```python
from build123d import *

# Parameters (mm, degrees)
CUT_EXTRUDE1_DEPTH      = 164.536310953
CUT_EXTRUDE1_DEPTH_BACK = 164.536310953
SKETCH2_R               = 6.05
SCALE1_SCALE            = 0.25


with BuildPart() as part:
    # Sketch1 → Revolve1 (revolve)
    with BuildSketch(Plane(origin=(0, 0, 0), x_dir=(0, 0, -1), z_dir=(1, 0, 0))):
        Polygon((-60, -15.260894059), (-60, -94.260894059), (-101.25, -94.260894059), (-101.25, -107.260894059), (-101.25, -115.260894059), (-54, -115.260894059), (-54, -94.260894059), (-34.1, -94.260894059), (-30, -94.160894059), (-30, -36.260894059), (-54, -36.260894059), (-54, -15.260894059), align=None)
    revolve(axis=Axis((0, 150, 0), (0, -1, 0)))

    # Sketch2 → Cut-Extrude1 (cut, two sides: drawn at the far end of the back side and taken through both)
    with BuildSketch(Plane(origin=(0, -94.260894059, 0), x_dir=(1, 0, 0), z_dir=(0, 1, 0)).offset(-CUT_EXTRUDE1_DEPTH_BACK)):
        with Locations(Location((0, 90, 0), (0, 0, 270))):
            Circle(SKETCH2_R)
        with Locations(Location((63.639610307, 63.639610307, 0), (0, 0, 270))):
            Circle(SKETCH2_R)
        with Locations(Location((90, 0, 0), (0, 0, 270))):
            Circle(SKETCH2_R)
        with Locations(Location((63.639610307, -63.639610307, 0), (0, 0, 270))):
            Circle(SKETCH2_R)
        with Locations(Location((0, -90, 0), (0, 0, 270))):
            Circle(SKETCH2_R)
        with Locations(Location((-63.639610307, -63.639610307, 0), (0, 0, 270))):
            Circle(SKETCH2_R)
        with Locations(Location((-90, 0, 0), (0, 0, 270))):
            Circle(SKETCH2_R)
        with Locations(Location((-63.639610307, 63.639610307, 0), (0, 0, 270))):
            Circle(SKETCH2_R)
    extrude(amount=CUT_EXTRUDE1_DEPTH + CUT_EXTRUDE1_DEPTH_BACK, mode=Mode.SUBTRACT)


with BuildPart() as part_1:
    # Scale1: scaled about (0, -81.802293933, 0)
    add(part.part.scale(SCALE1_SCALE).moved(Location((0, -61.35172045, 0))))


solid = part_1.part
```
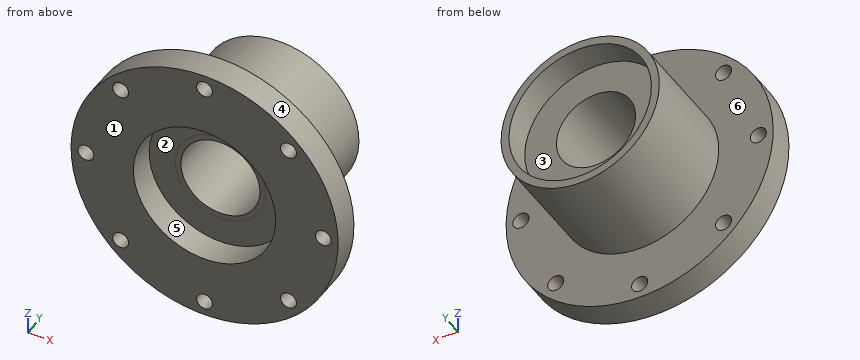
Verification items for the finished model (mm, model axes). Face numbers are marked on the shaded views. A direction names the side the tool comes from. Give positions to 0.01 mm unless a question says otherwise; leave off trailing zeros. Loops run counter-clockwise (first coordinate to the right, second up) from the corner with the lowest first, then second, coordinate; pieces in that order, holes last. Notation, with made-up numbers: M 71,84 L 104,84 A22 cw 104,96 Z; hole C -5,-13 d3. An arc over 180 degrees is marked long. One line per question, with ' | ' between items.
Item 1: Depth check by flat-ended pin: P1, Ø1, axis at y = -83.5, z = -10, coming from the -X side; P2, Ø1, axis at x = -1, z = -11, coming from the +Y side; P3, Ø3.5, axis at x = -15.91, z = 15.91, coming from the +Y side; P4, Ø3, axis at x = 4, z = 15, coming from the +Y side. Enter the tip coordinate at first touch or a pass-through.
Completed:
P1: stops at x = -11.61 | P2: stops at y = -70.42 | P3: stops at y = -84.92 | P4: stops at y = -65.17
Item 2: Section check D-D, the plane z = 22.5. Record the cut outline in (x, y), plus the area to 3 significant figures.
Completed:
outline: M -11.6,-90.17 L -1.51,-90.17 L -1.51,-84.92 L -11.6,-84.92 Z; M 1.51,-90.17 L 11.6,-90.17 L 11.6,-84.92 L 1.51,-84.92 Z | area: 106 mm^2
Item 3: Section check C-C, the plane y = -81. Record the cut outline in (x, z), plus the area to 3 significant figures.
Completed:
outline: C 0,0 d30; hole C 0,0 d15 | area: 530 mm^2
Item 4: Tool access check on the marked faces 1, 2 and 3. Record the directions out of +Z, -Z, +X, -X, +Y, -Y that give a thin tool (end or side, any length) a straight path to the whole face; none if there is none.
Completed:
face 1: +Z, -Z, +X, -X, -Y | face 2: -Y | face 3: +Y
Item 5: Section check B-B, the plane x = 22.5. Record the cut outline in (y, z), plus the area to 3 significant figures.
Completed:
outline: M -90.17,-11.6 L -84.92,-11.6 L -84.92,-1.51 L -90.17,-1.51 Z; M -90.17,1.51 L -84.92,1.51 L -84.92,11.6 L -90.17,11.6 Z | area: 106 mm^2
Item 6: Section check A-A, the plane x = 0. State how many separate pieces and enclosed holes the cut face has, plus the area to 3 significant figures.
Completed:
separate pieces: 4 | enclosed holes: 0 | area: 325 mm^2
Item 7: Draft check along X on the marked faces 4, 5 and 6. Enter one of: +X half, -X half, draft (parallel to the pull), parting line (faces both ways), or undercut.
Completed:
face 4: parting line | face 5: undercut | face 6: draft
Item 8: Thickness scan on line 1 (Z direction, x = 0, y = -87.35); line 2 (Z direction, x = 0, y = -67.6). Record the ranges inside material, lowest first. Write a range as [from, to].
Completed:
line 1: z = [-25.31, -24.01], [-20.99, -13.5], [13.5, 20.99], [24.01, 25.31] | line 2: z = [-15, -13.5], [13.5, 15]
